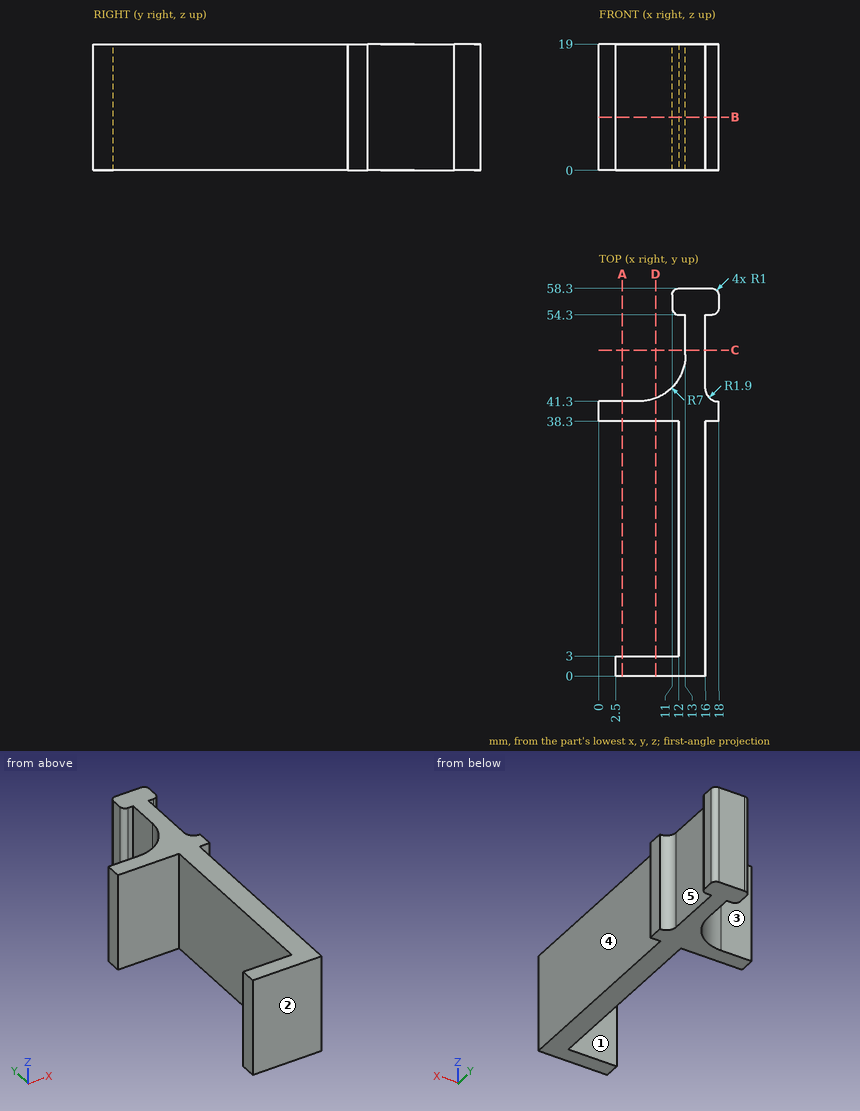
Job drawing, mm, ordinate dimensions from the low corner. One solid piece. A direction names the side the tool comes from. Coordinates: 2 decimals unless noted, no trailing zeros. Order: outer loops, then holes, each group sorted by start corner. A loop starts at its lowest first (then second) coordinate and runs counter-clockwise, first axis right, second up. Notation, with made-up numbers: (-18, 23.5) -> (-4, 23.5) arc R26 cw to (-4, 44.5) -> close; hole circle Ø4 at (25, -19). An arc over 180 degrees is marked (long way). Put each result on its own line as item: value. Start each with the question number.
(1) Band-saw the part on A-A (x = 3.5). Give the cut face in (y, z).
(2) Band-saw the part on D-D (x = 8.5). Give the cut face in (y, z), then the cut area to 3 significant figures.
(3) Band-saw the part on B-B (z = 8). Give the cut face in (x, y), then the cut area to 3 significant figures.
(4) Pin check, flat tips, straight feed: pin 1 Ø5 at (x, z) = (7.5, 12) entering from -Y; pin 2 Ø5 at (x, z) = (3, 8) entering from +Y; pin 3 Ø3 at (x, z) = (7, 6) entering from +Y; pin 4 Ø10 at (y, z) = (27.5, 16) entering from +X. Stop position of each tip, or through.
(5) Probe line 1 along Y through (x, z) = (4.5, 14.25); line 2 along X through (y, z) = (15, 18); line 3 along X through (y, z) = (51.5, 7.5). List the from-to ranges inside material, lowest first. Write a range as [from, to].
(6) Which spindle directions (+Z, -Z, +X, -X, +Y, -Y) get a long thin tool onto all of the face, cutting with end or side? Do the marked faces 1, 2, 3, 4 and 5. Say none if no direction does.
(7) Band-saw the part on C-C (y = 49). Give the cut face in (x, z), then the cut area to 3 significant figures.
Determined:
1. outline: (0, 0) -> (3, 0) -> (3, 19) -> (0, 19) -> close; (38.3, 0) -> (41.3, 0) -> (41.3, 19) -> (38.3, 19) -> close
2. outline: (0, 0) -> (3, 0) -> (3, 19) -> (0, 19) -> close; (38.3, 0) -> (41.76, 0) -> (41.76, 19) -> (38.3, 19) -> close
2. area: 123 mm²
3. outline: (0, 38.3) -> (12, 38.3) -> (12, 3) -> (2.5, 3) -> (2.5, 0) -> (16, 0) -> (16, 38.3) -> (18, 38.3) -> (18, 41.3) -> (17.9, 41.3) arc R1.9 cw to (16, 43.2) -> (16, 54.3) -> (17, 54.3) arc R1 ccw to (18, 55.3) -> (18, 57.3) arc R1 ccw to (17, 58.3) -> (12, 58.3) arc R1 ccw to (11, 57.3) -> (11, 55.3) arc R1 ccw to (12, 54.3) -> (13, 54.3) -> (13, 48.3) arc R7 cw to (6, 41.3) -> (0, 41.3) -> close
3. area: 313 mm²
4. pin 1: stops at y = 0
4. pin 2: stops at y = 41.3
4. pin 3: stops at y = 41.76
4. pin 4: stops at x = 16
5. line 1: y = [0, 3], [38.3, 41.3]
5. line 2: x = [12, 16]
5. line 3: x = [13, 16]
6. face 1: +Z, -Z, -X
6. face 2: +Z, -Z, +X, -X, -Y
6. face 3: +Z, -Z, -X, +Y
6. face 4: +Z, -Z, +X, -Y
6. face 5: +Z, -Z, +X
7. outline: (13, 0) -> (16, 0) -> (16, 19) -> (13, 19) -> close
7. area: 57.0 mm²
